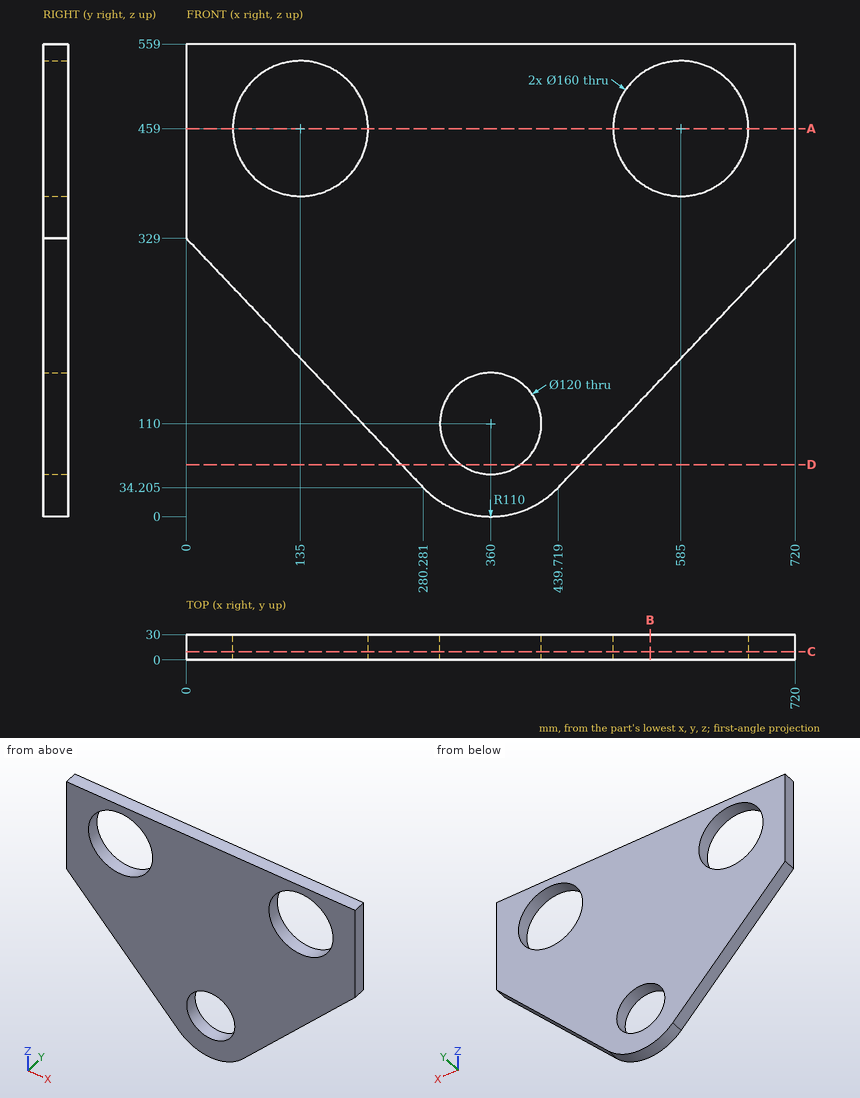
The figure shows three views and two pictorial views of one solid part (mm, origin at its lowest corner). Answer the questions. Give positions to 0.01 mm unless a question says otherwise; leave off trailing zeros. Loops run counter-clockwise (first coordinate to the right, second up) from the corner with the lowest first, then second, coordinate; pieces in that order, holes last. Notation, with made-up numbers: (-17, 42.5) -> (18, 42.5) arc R32 ccw to (18, 73.5) -> close; hole circle Ø1 at (-39, 85). An arc over 180 degrees is marked (long way). Use CSV: the item, a comma, the result in double quotes.
1. Flat-ended cylindrical pins translate along their axes: pin 1 Ø8 at (y, z) = (4.5, 209.5) entering from -X (1 decimal); pin 2 Ø2 at (y, z) = (19.5, 249) entering from +X; pin 3 Ø8 at (y, z) = (7, 146) entering from -X; pin 4 Ø12 at (x, z) = (464, 406.5) entering from -Y. Find the tip coordinate at first contact, or state that the pin passes through.
Found:
pin 1,"x = 109.8"
pin 2,"x = 644.89"
pin 3,"x = 170.19"
pin 4,"y = 0"
2. The part is cut by section B-B (x = 548.5). Write down the section's boundary in (y, z), then the cut area to 3 significant figures.
Found:
outline,"(0, 148.62) -> (30, 148.62) -> (30, 387.81) -> (0, 387.81) -> close; (0, 530.19) -> (30, 530.19) -> (30, 559) -> (0, 559) -> close"
area,"8,040 mm^2"
3. The part is cut by section A-A (z = 459). Write down the section's boundary in (x, y), then the cut area to 3 significant figures.
Found:
outline,"(0, 0) -> (55, 0) -> (55, 30) -> (0, 30) -> close; (215, 0) -> (505, 0) -> (505, 30) -> (215, 30) -> close; (665, 0) -> (720, 0) -> (720, 30) -> (665, 30) -> close"
area,"12,000 mm^2"
4. The part is cut by section C-C (y = 9.75). Write down the section's boundary in (x, z) (1 decimal).
Found:
outline,"(0, 329) -> (280.3, 34.2) arc R110 ccw to (439.7, 34.2) -> (720, 329) -> (720, 559) -> (0, 559) -> close; hole circle Ø160 at (135, 459); hole circle Ø120 at (360, 110); hole circle Ø160 at (585, 459)"
5. Straight lines are drawn through the part: line 1 (X direction, y = 2.75, z = 392.5) (1 decimal); line 2 (Z direction, x = 360, y = 8.25); line 3 (X direction, y = 15, z = 532) (1 decimal). For each, find the intervals that lie inside material, in ascending order.
Found:
line 1,"0 to 90.5, 179.5 to 540.5, 629.5 to 720"
line 2,"0 to 50, 170 to 559"
line 3,"0 to 102.3, 167.7 to 552.3, 617.7 to 720"
6. The part is cut by section D-D (z = 61.5). Write down the section's boundary in (x, y).
Found:
outline,"(254.33, 0) -> (324.68, 0) -> (324.68, 30) -> (254.33, 30) -> close; (395.32, 0) -> (465.67, 0) -> (465.67, 30) -> (395.32, 30) -> close"
